```python
from build123d import *

# Parameters (mm, degrees)
F1_DEPTH = 381
F3_DEPTH = 127
F5_DEPTH = 381


with BuildPart() as f1:
    # F0 (on Front) → F1 (new body, symmetric)
    with BuildSketch(Plane.XZ):
        with BuildLine():
            ThreePointArc((-174.625, -147.526504), (-228.6, 0), (-174.625, 147.526504))
            Line((-174.625, 147.526504), (-174.625, 152.4))
            ThreePointArc((-174.625, 152.4), (-231.775, 0), (-174.625, -152.4))
            Line((-174.625, -152.4), (-174.625, -147.526504))
        make_face()
    extrude(amount=F1_DEPTH, both=True)

    # F2 (on Front) → F3 (join, symmetric)
    with BuildSketch(Plane.XZ):
        Polygon((-226.20073, 88.459134), (-243.843385, -11.597334), (-237.339714, -12.744107), (-219.69706, 87.312361), align=None)
    extrude(amount=F3_DEPTH, both=True)

    # F4 (on Front) → F5 (join, symmetric)
    with BuildSketch(Plane.XZ):
        Polygon((-168.469529, -155.732401), (-163.286397, -151.639974), (-179.026501, -131.704851), (-184.209633, -135.797278), align=None)
    extrude(amount=F5_DEPTH, both=True)


solid = f1.part
```
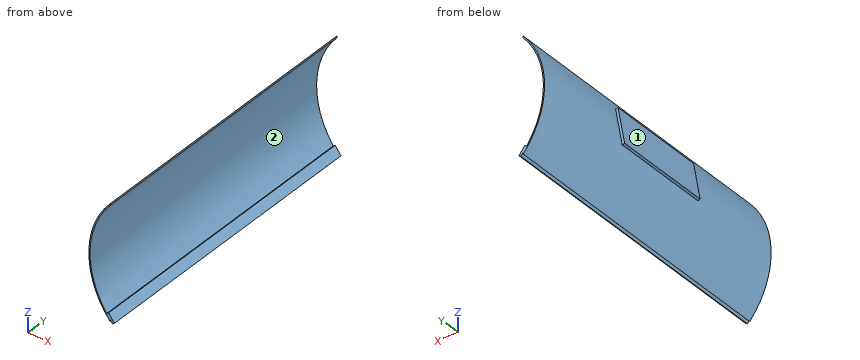
The model under review builds one solid part; all positions refer to its coordinate system, in mm. Face numbers are marked on the shaded views. Give positions to 0.01 mm unless a question says otherwise; leave off trailing zeros. Write each loop counter-clockwise with the first axis right and the second up, starting at its lowest first coordinate (ties: lowest second). Pieces come first, ordered by that corner, then holes. Notation, with made-up numbers: (17, 87) -> (46, 87) arc R19 cw to (46, 106) -> close; hole circle Ø5 at (74.25, 16). An arc over 180 degrees is marked (long way). Put each result on its own line as item: value.
(1) For pin 1 Ø2 at (y, z) = (-245, -36.5) entering from -X; pin 2 Ø6 at (x, y) = (-181, 267) entering from +Z; pin 3 Ø4 at (x, y) = (-182, 19.5) entering from -Z, all flat-tipped, find the tip position at first contact; note any pin that passes through.
Results are:
pin 1: x = -229.04
pin 2: z = 148.44
pin 3: z = -146.01
(2) We need section B-B, the plane x = -192. Give the boundary of the cut face in (y, z), and give its area (3 significant figures).
Results are:
outline: (-381, -129.83) -> (381, -129.83) -> (381, -124.07) -> (-381, -124.07) -> close; (-381, 124.07) -> (381, 124.07) -> (381, 129.83) -> (-381, 129.83) -> close
area: 8,770 mm²
(3) We need section C-C, the plane z = 11.5. Give the boundary of the cut face in (x, y).
Results are:
outline: (-239.77, -127) -> (-233.06, -127) -> (-233.06, 127) -> (-239.77, 127) -> close; (-231.49, -381) -> (-228.31, -381) -> (-228.31, 381) -> (-231.49, 381) -> close
(4) The part is to be moulded in two halves that separate along Z. For the marked faces 1 and 2, say which applies: pulls with the +Z half, pulls with the -Z half, needs draft (parallel to the pull), parting line crosses it, or undercut.
Results are:
face 1: pulls with the +Z half
face 2: undercut
(5) To check wall thickness, follow probe 1 along Z at (x, y) = (-207.5, -80); probe 2 along Z at (x, y) = (-211, -278); probe 3 along X at (y, z) = (-6.5, 0) (3 decimals). State the ranges of each line that lie inside material, in increasing order. Write a range as from..to.
Results are:
probe 1: -103.26..-95.93, 95.93..103.26
probe 2: -95.91..-87.96, 87.96..95.91
probe 3: -241.798..-235.093, -231.775..-228.6
